Could you check a few things on this model? Use its own coordinates, in mm. Coordinates: 2 decimals unless noted, no trailing zeros. Order: outer loops, then holes, each group sorted by start corner. A loop starts at its lowest first (then second) coordinate and runs counter-clockwise, first axis right, second up. Notation, with made-up numbers: (24.5, 81.5) -> (35.5, 81.5) arc R24 ccw to (35.5, 119.5) -> close; hole circle Ø11 at (-13, 24.25). An arc over 180 degrees is marked (long way). Use a Markdown table: item, result. Add a question column.
1) Thinking about a two-plate mould opening in Y: for faces 1 (the cylindrical face through (142.15, 143.373, 1.627)), 2 (the cylindrical face through (184.297, 183.986, 1.627)), 3 (the flat face through (122, 72, 3.3)), which applies, +Y half, -Y half, draft (parallel to the pull), parting line (faces both ways), or undercut?
2) If we section it at D-D (y = 70): Write out the boundary of the cut face in (x, z), plus the area to 3 significant figures.
3) If I drill on L1, parallel to Y at x = 140, z = 1.75; L2, parallel to Y at x = 170, z = 0.85; L3, parallel to X at y = -2, z = 0.95, over which ranges is the centre line in solid material (lowest first)? Write a range as [from, to].
4) Will this pin go through, and if not, where does the flat tip stop? pin 1 Ø5 at (x, y) = (140, 140) entering from +Z.
5) If we section it at A-A (x = 140): Write out the boundary of the cut face in (y, z).
6) If we section it at C-C (z = 2.8): Give the number of separate pieces and of enclosed holes in the cut face, plus the area to 3 significant figures.
```python
from build123d import *

# Parameters (mm, degrees)
F0_R     = 5
F0_R_2   = 4
F0_R_3   = 45
F1_DEPTH = 3.3


with BuildPart() as f1:
    # F0 (on Top) → F1 (new body)
    with BuildSketch(Plane.XY):
        with BuildLine():
            Line((170, 190), (-30, 190))
            ThreePointArc((-30, 190), (-44.142136, 184.142136), (-50, 170))
            Line((-50, 170), (-50, -30))
            ThreePointArc((-50, -30), (-44.142136, -44.142136), (-30, -50))
            Line((-30, -50), (170, -50))
            ThreePointArc((170, -50), (184.142136, -44.142136), (190, -30))
            Line((190, -30), (190, 170))
            ThreePointArc((190, 170), (184.142136, 184.142136), (170, 190))
        make_face()
        with Locations((-30, -30)):
            Circle(F0_R, mode=Mode.SUBTRACT)
        Circle(F0_R_2, mode=Mode.SUBTRACT)
        with Locations((170, -30)):
            Circle(F0_R, mode=Mode.SUBTRACT)
        with Locations((140, 0)):
            Circle(F0_R_2, mode=Mode.SUBTRACT)
        with Locations((0, 140)):
            Circle(F0_R_2, mode=Mode.SUBTRACT)
        with Locations((-30, 170)):
            Circle(F0_R, mode=Mode.SUBTRACT)
        with Locations((70, 70)):
            Circle(F0_R_3, mode=Mode.SUBTRACT)
        with Locations((140, 140)):
            Circle(F0_R_2, mode=Mode.SUBTRACT)
        with Locations((170, 170)):
            Circle(F0_R, mode=Mode.SUBTRACT)
    extrude(amount=F1_DEPTH)


solid = f1.part
```
Answer sheet:
| question | item | result |
|---|---|---|
| 1 | face 1 | undercut |
| 1 | face 2 | +Y half |
| 1 | face 3 | draft |
| 2 | outline | (-50, 0) -> (25, 0) -> (25, 3.3) -> (-50, 3.3) -> close; (115, 0) -> (190, 0) -> (190, 3.3) -> (115, 3.3) -> close |
| 2 | area | 495 mm2 |
| 3 | L1 | [-50, -4], [4, 136], [144, 190] |
| 3 | L2 | [-50, -35], [-25, 165], [175, 190] |
| 3 | L3 | [-50, -3.46], [3.46, 136.54], [143.46, 190] |
| 4 | pin 1 | through |
| 5 | outline | (-50, 0) -> (-4, 0) -> (-4, 3.3) -> (-50, 3.3) -> close; (4, 0) -> (136, 0) -> (136, 3.3) -> (4, 3.3) -> close; (144, 0) -> (190, 0) -> (190, 3.3) -> (144, 3.3) -> close |
| 6 | separate pieces | 1 |
| 6 | enclosed holes | 9 |
| 6 | area | 50,400 mm2 |
